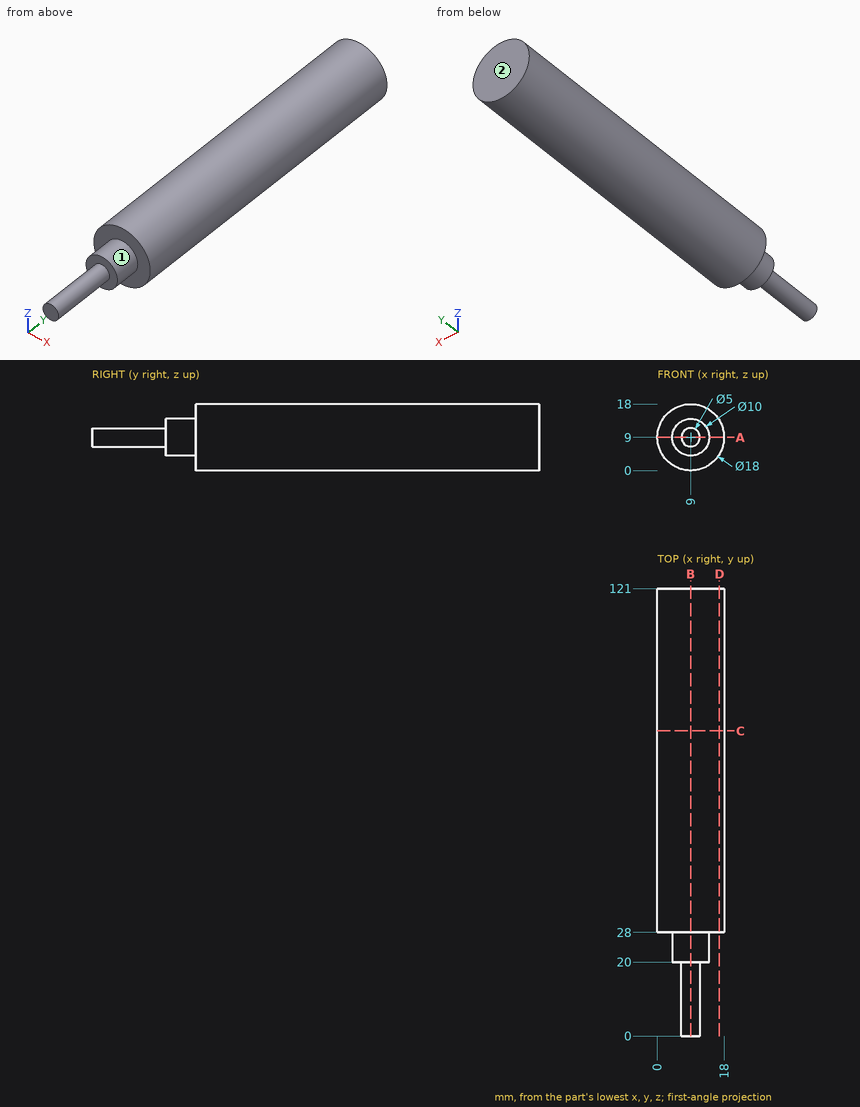
Job drawing, mm, ordinate dimensions from the low corner. One solid piece. A direction names the side the tool comes from. Round coordinates to 2 decimals unless told otherwise and drop trailing zeros. Write each loop counter-clockwise with the first axis right and the second up, starting at its lowest first coordinate (ties: lowest second). Pieces come first, ordered by that corner, then holes. Notation, with made-up numbers: M 26,0 L 73,0 A30 cw 73,25 Z; hole C -11.5,-19.5 d3. An arc over 180 degrees is marked long. Return JSON: item names as keys, results as strings. Group by question number.
(1) Saw through at A-A on z = 9. Write the cut outline in (x, y), then the cut area to 3 significant figures.
(2) Saw through at D-D on x = 16.75. Write the cut outline in (y, z), then the cut area to 3 significant figures.
(3) Drill centre lines: probe 1 along Y at (x, z) = (1, 6.5); probe 2 along Y at (x, z) = (4.25, 8.5); probe 3 along Z at (x, y) = (9.25, 27). Where is each one in solid material? Low to high.
(4) Pin check, flat tips, straight feed: pin 1 Ø10 at (x, z) = (3, 12) entering from -Y; pin 2 Ø1.5 at (y, z) = (95, 4.5) entering from -X; pin 3 Ø6 at (y, z) = (58, 5) entering from +X; pin 4 Ø2 at (y, z) = (13, 13.5) entering from +X. Stop position of each tip, or through.
(5) Saw through at C-C on y = 82.5. Write the cut outline in (x, z).
(6) Which spindle directions (+Z, -Z, +X, -X, +Y, -Y) get a long thin tool onto all of the face, cutting with end or side? Do the marked faces 1 and 2. Say none if no direction does.
(7) Saw through at B-B on x = 9. Write the cut outline in (y, z).
Returned:
{
 "1": {"outline": "M 0,28 L 4,28 L 4,20 L 6.5,20 L 6.5,0 L 11.5,0 L 11.5,20 L 14,20 L 14,28 L 18,28 L 18,121 L 0,121 Z", "area": "1,850 mm²"},
 "2": {"outline": "M 28,4.42 L 121,4.42 L 121,13.58 L 28,13.58 Z", "area": "851 mm²"},
 "3": {"probe 1": "28 to 121", "probe 2": "20 to 121", "probe 3": "4.01 to 13.99"},
 "4": {"pin 1": "y = 0", "pin 2": "x = 0.82", "pin 3": "x = 17.94", "pin 4": "through"},
 "5": {"outline": "C 9,9 d18"},
 "6": {"face 1": "-Y", "face 2": "+Z, -Z, +X, -X, +Y"},
 "7": {"outline": "M 0,6.5 L 20,6.5 L 20,4 L 28,4 L 28,0 L 121,0 L 121,18 L 28,18 L 28,14 L 20,14 L 20,11.5 L 0,11.5 Z"}
}
